Verification items for the finished model (mm, model axes). Give positions to 0.01 mm unless a question says otherwise; leave off trailing zeros. Write each loop counter-clockwise with the first axis right and the second up, starting at its lowest first coordinate (ties: lowest second). Pieces come first, ordered by that corner, then holes. Notation, with made-up numbers: (70.5, -20) -> (85.5, -20) arc R26 cw to (85.5, 12) -> close; hole circle Ø5 at (57.5, 19). An arc over 180 degrees is marked (long way). Answer as CSV lines item,"result".
```python
from build123d import *

# Parameters (mm, degrees)
F0_W          = 30
F0_H          = 57
F1_DEPTH      = 5
F1_DEPTH_BACK = 5
F2_R          = 5
F3_R          = 2.074
F4_DEPTH      = 10.001
F5_SIZE       = 2


with BuildPart() as f1:
    # F0 (on Front) → F1 (new body, two sides)
    with BuildSketch(Plane.XZ) as f1_sk:
        Rectangle(F0_W, F0_H)
    extrude(amount=F1_DEPTH)
    extrude(f1_sk.sketch, amount=-F1_DEPTH_BACK)

    # F2
    f2_edges = [f1.edges().sort_by_distance(p)[0] for p in [
        (-15, 0, 28.5),
        (15, 0, 28.5),
        (-15, 0, -28.5),
        (15, 0, -28.5),
    ]]
    fillet(f2_edges, radius=F2_R)

    # F3 (on face) → F4 (cut, through all)
    with BuildSketch(Plane.XZ.offset(5)):
        with Locations((-10, 23.5)):
            Circle(F3_R)
        with Locations((10, 23.5)):
            Circle(F3_R)
        with Locations((-10, -23.5)):
            Circle(F3_R)
        with Locations((10, -23.5)):
            Circle(F3_R)
    extrude(amount=-F4_DEPTH, mode=Mode.SUBTRACT)

    # F5
    f5_edges = [f1.edges().sort_by_distance(p)[0] for p in [
        (-12.074, -5, 23.5),
        (7.926, -5, 23.5),
        (-12.074, -5, -23.5),
        (7.926, -5, -23.5),
    ]]
    chamfer(f5_edges, length=F5_SIZE)


solid = f1.part
```
1) Scan lines: line 1 along Z through (x, y) = (10, 0); line 2 along X through (y, z) = (-1, -25); line 3 along Z through (x, y) = (11.5, 3.75). Record each from-to range of solid material in increasing order.
Reported:
line 1,"-28.5 to -25.57, -21.43 to 21.43, 25.57 to 28.5"
line 2,"-14.77 to -11.43, -8.57 to 8.57, 11.43 to 14.77"
line 3,"-28.27 to -24.93, -22.07 to 22.07, 24.93 to 28.27"
2) Draft check along X on faces 1 (the cylindrical face through (9.73, 0.944, -21.444)), 2 (the cylindrical face through (-13.57, -0.07, -27)), 3 (the flat face through (15, 0, 0)). Enter one of: +X half, -X half, draft (parallel to the pull), parting line (faces both ways), or undercut.
Reported:
face 1,"undercut"
face 2,"-X half"
face 3,"+X half"
3) Section check A-A (y = -0.5). Record the boundary of the cut face in (x, z), and give its area (3 significant figures).
Reported:
outline,"(-15, -23.5) arc R5 ccw to (-10, -28.5) -> (10, -28.5) arc R5 ccw to (15, -23.5) -> (15, 23.5) arc R5 ccw to (10, 28.5) -> (-10, 28.5) arc R5 ccw to (-15, 23.5) -> close; hole circle Ø4.15 at (-10, -23.5); hole circle Ø4.15 at (-10, 23.5); hole circle Ø4.15 at (10, -23.5); hole circle Ø4.15 at (10, 23.5)"
area,"1,630 mm²"
4) Depth check by flat-ended pin: pin 1 (2 mm diameter, centred on x = 12, y = -2, fed in from +Z); pin 2 (5 mm diameter, centred on x = -10, z = 23.5, fed in from -Y); pin 3 (5.5 mm diameter, centred on x = 10, z = 23.5, fed in from -Y). Enter the tip coordinate at first touch or a pass-through.
Reported:
pin 1,"z = 28.4"
pin 2,"y = -3.43"
pin 3,"y = -3.68"
